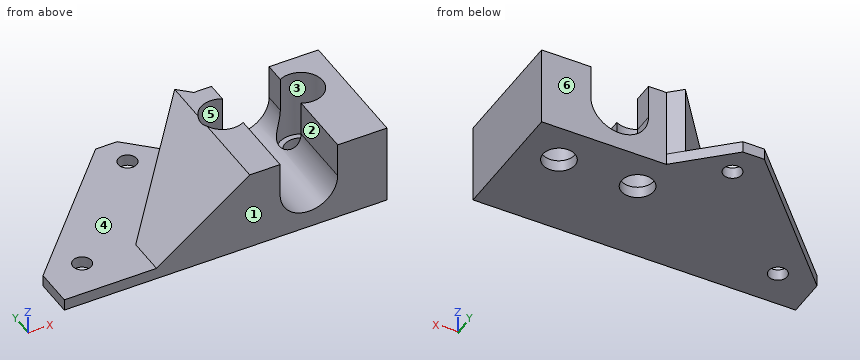
```python
from build123d import *

# Parameters (mm, degrees)
BOSS_EXTRUDE1_DEPTH     = 2
SKETCH3_R               = 1.6
SKETCH3_R_2             = 2.8
CUT_EXTRUDE1_DEPTH      = 2
SKETCH5_R               = 3.75
BOSS_EXTRUDE2_DEPTH     = 12
CUT_EXTRUDE2_DEPTH      = 41.633693803
CUT_EXTRUDE3_DEPTH      = 41.633693891
CUT_EXTRUDE3_DEPTH_BACK = 41.633693891


with BuildPart() as part:
    # Sketch2 → Boss-Extrude1 (new body)
    with BuildSketch(Plane.XY):
        Polygon((-24.662569153, 7.22803975), (-2.803398565, 30.477324023), (0.929669822, 30.477324023), (9.704320922, 22.227324023), (31.337430847, 22.227324023), (31.337430847, 0.477324023), (-24.662569153, 0.477324023), align=None)
    extrude(amount=BOSS_EXTRUDE1_DEPTH)

    # Sketch3 → Cut-Extrude1 (cut)
    with BuildSketch(Plane.XY.offset(2)):
        with Locations((-0.012297753, 25.477324023)):
            Circle(SKETCH3_R)
        with Locations((-18.012297753, 6.977324023)):
            Circle(SKETCH3_R)
        with Locations((10.987702247, 15.477324023)):
            Circle(SKETCH3_R_2)
        with Locations((24.587430847, 15.391405477)):
            Circle(SKETCH3_R_2)
    extrude(amount=-CUT_EXTRUDE1_DEPTH, mode=Mode.SUBTRACT)

    # Sketch5 → Boss-Extrude2 (add)
    with BuildSketch(Plane.XY.offset(2)):
        Polygon((-8.662569153, 7.072030866), (7.518665156, 24.282295767), (9.704320922, 22.227324023), (31.337430847, 22.227324023), (31.337430847, 3.477324023), (31.337430847, 0.477324023), (-8.662569153, 0.477324023), align=None)
        with Locations((10.987702247, 15.477324023)):
            Circle(SKETCH5_R, mode=Mode.SUBTRACT)
        with Locations((24.587430847, 15.391405477)):
            Circle(SKETCH5_R, mode=Mode.SUBTRACT)
    extrude(amount=BOSS_EXTRUDE2_DEPTH)

    # Sketch10 → Cut-Extrude2 (cut, through all)
    with BuildSketch(Plane(origin=(0, 22.227324023, 0), x_dir=(1, 0, 0), z_dir=(0, 1, 0))):
        with BuildLine():
            Line((12.787295144, -14), (12.787295144, -8))
            ThreePointArc((12.787295144, -8), (17.787295144, -3), (22.787295144, -8))
            Line((22.787295144, -8), (22.787295144, -14))
            ThreePointArc((22.787295144, -14), (17.787295144, -19), (12.787295144, -14))
        make_face()
    extrude(amount=-CUT_EXTRUDE2_DEPTH, mode=Mode.SUBTRACT)

    # Sketch11 → Cut-Extrude3 (cut, two sides: drawn at the far end of the back side and taken through both)
    with BuildSketch(Plane(origin=(0, 22.227324023, 0), x_dir=(1, 0, 0), z_dir=(0, 1, 0)).offset(-CUT_EXTRUDE3_DEPTH_BACK)):
        Polygon((-8.662569153, -2), (7.518665156, -14), (-8.662569153, -14), align=None)
    extrude(amount=CUT_EXTRUDE3_DEPTH + CUT_EXTRUDE3_DEPTH_BACK, mode=Mode.SUBTRACT)


solid = part.part
```
Work out the finished part from the listing and answer in its coordinate system (mm). Face numbers are marked on the shaded views. A direction names the side the tool comes from. Coordinates: 2 decimals unless noted, no trailing zeros. Order: outer loops, then holes, each group sorted by start corner. A loop starts at its lowest first (then second) coordinate and runs counter-clockwise, first axis right, second up. Notation, with made-up numbers: M -16.5,31 L 7.5,31 A6 cw 7.5,37 Z; hole C -27.5,66.25 d6. An arc over 180 degrees is marked long. Use CSV: the item, a comma, the result in double quotes.
1) Section B-B on y = 10 is taken. Write down the section's boundary in (x, z).
Worked out:
outline,"M -22.06,0 L 31.34,0 L 31.34,14 L 22.79,14 L 22.79,8 A5 cw 12.79,8 L 12.79,14 L 7.52,14 L -5.91,4.04 L -5.91,2 L -22.06,2 Z"
2) Determine the mould class of the marked faces 1, 2 and 3 for opening direction Y: released by +Y, released by -Y, zero draft, split by the parting line, or undercut.
Worked out:
face 1,"released by -Y"
face 2,"zero draft"
face 3,"undercut"
3) For the marked faces 4, 5 and 6, determine the directions among +Z, -Z, +X, -X, +Y, -Y from which every point of the face is accessible in a straight line to the end or side of a thin tool.
Worked out:
face 4,"+Z, -X, +Y"
face 5,"+Z"
face 6,"+Z, -Z, +X, +Y"
4) Section A-A on z = 6.5 is taken. Write down the section's boundary in (x, y), plus the area to 3 significant figures.
Worked out:
outline,"M -2.59,0.48 L 13.02,0.48 L 13.02,12.32 A3.75 cw long 13.02,18.63 L 13.02,22.23 L 9.7,22.23 L 7.52,24.28 L -2.59,13.53 Z; M 22.56,0.48 L 31.34,0.48 L 31.34,22.23 L 22.56,22.23 L 22.56,18.54 A3.75 cw long 22.56,12.24 Z"
area,"426 mm^2"
5) Consider line 1 (X direction, y = 19.5, z = 3.75); line 2 (Z direction, x = -8, y = 23); line 3 (Y direction, x = 19.5, z = 2.5). Determine where each line is inside the solid, lowest interval first. Write a range as [from, to].
Worked out:
line 1,"x = [3.02, 15.15], [20.42, 31.34]"
line 2,"z = [0, 2]"
line 3,"y = [0.48, 22.23]"
6) Flat-ended cylindrical pins translate along their axes: pin 1 Ø7.5 at (x, y) = (10.99, 15.48) entering from -Z; pin 2 Ø6 at (x, y) = (-3, 12.5) entering from +Z; pin 3 Ø5 at (y, z) = (5, 9.5) entering from -X; pin 4 Ø2 at (x, y) = (11, 16) entering from +Z. Find the tip coordinate at first contact, or state that the pin passes through.
Worked out:
pin 1,"stops at z = 0"
pin 2,"stops at z = 8.42"
pin 3,"stops at x = -1.92"
pin 4,"passes through"
